from build123d import *

# Parameters (mm, degrees)
SKETCH_1_W          = 40
SKETCH_1_H          = 20
SKETCH_1_R          = 1
EXTRUDE_1_DEPTH     = 40
FILLET_1_R          = 1.5
SKETCH_3_R          = 6.5
EXTRUDE_3_DEPTH     = 1.4
EXTRUDE_START       = 1.4
SKETCH_4_R          = 6.5
EXTRUDE_4_DEPTH     = 1.4
SKETCH_6_R          = 3
EXTRUDE_6_DEPTH     = 4
SKETCH_7_W          = 8
SKETCH_7_H          = 4.7
CUT_EXTRUDE_1_DEPTH = 3
SKETCH_8_W          = 4.7
SKETCH_8_H          = 8
CUT_EXTRUDE_2_DEPTH = 3


with BuildPart() as part:
    # 草图1 → 凸台-拉伸1 (new body)
    with BuildSketch(Plane.XY):
        with Locations((-36.575311459, 110.529011993)):
            Rectangle(SKETCH_1_W, SKETCH_1_H)
        with Locations((-54.575311459, 118.529011993)):
            Circle(SKETCH_1_R, mode=Mode.SUBTRACT)
        with Locations((-54.575311459, 102.529011993)):
            Circle(SKETCH_1_R, mode=Mode.SUBTRACT)
        with Locations((-18.575311459, 102.529011993)):
            Circle(SKETCH_1_R, mode=Mode.SUBTRACT)
        with Locations((-18.575311459, 118.529011993)):
            Circle(SKETCH_1_R, mode=Mode.SUBTRACT)
    extrude(amount=EXTRUDE_1_DEPTH)

    # 圆角1
    fillet_1_edges = [part.edges().sort_by_distance(p)[0] for p in [
        (-16.575311459, 100.529011993, 20),
        (-56.575311459, 100.529011993, 20),
        (-56.575311459, 120.529011993, 20),
        (-16.575311459, 120.529011993, 20),
    ]]
    fillet(fillet_1_edges, radius=FILLET_1_R)

    # 草图3 → 凸台-拉伸3 (add)
    with BuildSketch(Plane.XY.offset(40)):
        with Locations((-46.775311459, 110.529011993)):
            Circle(SKETCH_3_R)
    extrude(amount=EXTRUDE_3_DEPTH)

    # 草图4 → 凸台-拉伸4 (add)
    with BuildSketch(Plane(origin=(0, 0, 0), x_dir=(-1, 0, 0), z_dir=(0, 0, -1)).offset(EXTRUDE_START)):
        with Locations(Location((46.775311459, 110.529011993, 0), (0, 0, 180))):
            Circle(SKETCH_4_R)
    extrude(amount=-EXTRUDE_4_DEPTH)

    # 草图6 → 凸台-拉伸6 (add)
    with BuildSketch(Plane.XY.offset(41.4)):
        with Locations((-46.775311459, 110.529011993)):
            Circle(SKETCH_6_R)
    extrude(amount=EXTRUDE_6_DEPTH)

    # 草图7 → 切除-拉伸1 (cut)
    with BuildSketch(Plane.XZ.offset(-100.529011993)):
        with Locations((-42.575311459, 8.35)):
            Rectangle(SKETCH_7_W, SKETCH_7_H)
    cut_extrude_1 = extrude(amount=-CUT_EXTRUDE_1_DEPTH, mode=Mode.SUBTRACT)

    # 镜向1: 切除-拉伸1 across plane
    add(cut_extrude_1.mirror(Plane(origin=(0, 110.529011993, 0), x_dir=(0, 0, 1), z_dir=(0, -1, 0))), mode=Mode.SUBTRACT)

    # 草图8 → 切除-拉伸2 (cut)
    with BuildSketch(Plane.ZY.offset(56.575311459)):
        with Locations((8.35, 110.529011993)):
            Rectangle(SKETCH_8_W, SKETCH_8_H)
    extrude(amount=-CUT_EXTRUDE_2_DEPTH, mode=Mode.SUBTRACT)


solid = part.part
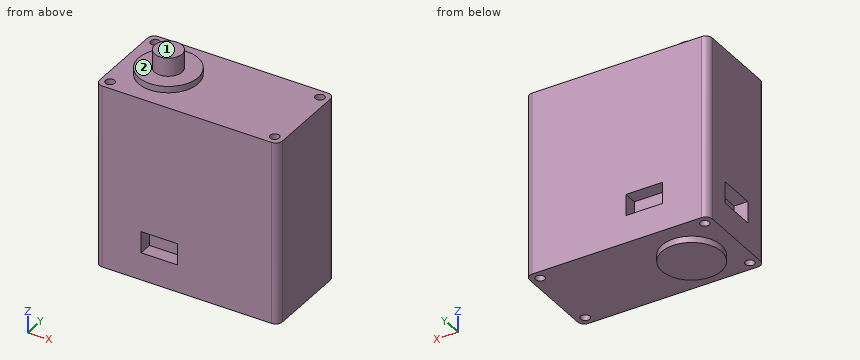
Read the model definition and answer for the solid it produces. Units are mm, in the model's axes. Face numbers are marked on the shaded views. A direction names the side the tool comes from. Give positions to 0.01 mm unless a question says otherwise; leave off trailing zeros. Loops run counter-clockwise (first coordinate to the right, second up) from the corner with the lowest first, then second, coordinate; pieces in that order, holes last. Notation, with made-up numbers: (-5.75, -34.75) -> (11.25, -34.75) arc R20 cw to (11.25, 4.25) -> close; hole circle Ø10 at (84, 61). An arc over 180 degrees is marked (long way). Use a Markdown table: item, result.
Q1. Section D-D, the plane z = 8 is taken. Determine the outline of the cut face in (x, y).
Solved:
| item | result |
|---|---|
| outline | (-56.58, 102.03) arc R1.5 ccw to (-55.08, 100.53) -> (-46.58, 100.53) -> (-46.58, 103.53) -> (-38.58, 103.53) -> (-38.58, 100.53) -> (-18.08, 100.53) arc R1.5 ccw to (-16.58, 102.03) -> (-16.58, 119.03) arc R1.5 ccw to (-18.08, 120.53) -> (-38.58, 120.53) -> (-38.58, 117.53) -> (-46.58, 117.53) -> (-46.58, 120.53) -> (-55.08, 120.53) arc R1.5 ccw to (-56.58, 119.03) -> (-56.58, 114.53) -> (-53.58, 114.53) -> (-53.58, 106.53) -> (-56.58, 106.53) -> close; hole circle Ø2 at (-54.58, 102.53); hole circle Ø2 at (-54.58, 118.53); hole circle Ø2 at (-18.58, 102.53); hole circle Ø2 at (-18.58, 118.53) |
Q2. Section A-A, the plane z = 34 is taken. Determine the outline of the cut face in (x, y), then the cut area to 4 significant figures.
Solved:
| item | result |
|---|---|
| outline | (-56.58, 102.03) arc R1.5 ccw to (-55.08, 100.53) -> (-18.08, 100.53) arc R1.5 ccw to (-16.58, 102.03) -> (-16.58, 119.03) arc R1.5 ccw to (-18.08, 120.53) -> (-55.08, 120.53) arc R1.5 ccw to (-56.58, 119.03) -> close; hole circle Ø2 at (-54.58, 102.53); hole circle Ø2 at (-54.58, 118.53); hole circle Ø2 at (-18.58, 102.53); hole circle Ø2 at (-18.58, 118.53) |
| area | 785.5 mm^2 |
Q3. Section B-B, the plane x = -48 is taken. Determine the outline of the cut face in (y, z), then the cut area to 3 significant figures.
Solved:
| item | result |
|---|---|
| outline | (100.53, 0) -> (104.15, 0) -> (104.15, -1.4) -> (116.91, -1.4) -> (116.91, 0) -> (120.53, 0) -> (120.53, 40) -> (116.91, 40) -> (116.91, 41.4) -> (113.27, 41.4) -> (113.27, 45.4) -> (107.79, 45.4) -> (107.79, 41.4) -> (104.15, 41.4) -> (104.15, 40) -> (100.53, 40) -> close |
| area | 858 mm^2 |
Q4. Each of these flat-tipped pins is pushed along its axis until it touches: pin 1 (3.5 mm diameter, centred on x = -55.5, y = 109.5, fed in from +Z); pin 2 (3.5 mm diameter, centred on x = -41, y = 119, fed in from -Z); pin 3 (4 mm diameter, centred on x = -44.5, z = 8.5, fed in from -Y); pin 4 (10.5 mm diameter, centred on x = -45, y = 113.5, fed in from +Z). Where does it stop, or does it pass through?
Solved:
| item | result |
|---|---|
| pin 1 | stops at z = 40 |
| pin 2 | stops at z = 0 |
| pin 3 | stops at y = 103.53 |
| pin 4 | stops at z = 45.4 |
Q5. Find the intervals of material crossed by line 1 along X through (y, z) = (118.5, 7); line 2 along Y through (x, z) = (-54, 7.5); line 3 along Z through (x, y) = (-23.5, 109.25), in increasing order.
Solved:
| item | result |
|---|---|
| line 1 | x = -56.58 to -55.57, -53.58 to -46.58, -38.58 to -19.57, -17.58 to -16.58 |
| line 2 | y = 100.53 to 101.71, 103.35 to 106.53, 114.53 to 117.71, 119.35 to 120.53 |
| line 3 | z = 0 to 40 |
Q6. A tool of negligible diameter and unlimited length cuts with its end or side. For the marked faces 1 and 2, from which of +Z, -Z, +X, -X, +Y, -Y can it reach the whole face along a straight path? Write none if from no direction.
Solved:
| item | result |
|---|---|
| face 1 | +Z, +X, -X, +Y, -Y |
| face 2 | +Z |
Q7. Section C-C, the plane y = 112.5 is taken. Determine the outline of the cut face in (x, z), then the cut area to 3 significant figures.
Solved:
| item | result |
|---|---|
| outline | (-56.58, 0) -> (-52.97, 0) -> (-52.97, -1.4) -> (-40.58, -1.4) -> (-40.58, 0) -> (-16.58, 0) -> (-16.58, 40) -> (-40.58, 40) -> (-40.58, 41.4) -> (-44.51, 41.4) -> (-44.51, 45.4) -> (-49.04, 45.4) -> (-49.04, 41.4) -> (-52.97, 41.4) -> (-52.97, 40) -> (-56.58, 40) -> (-56.58, 10.7) -> (-53.58, 10.7) -> (-53.58, 6) -> (-56.58, 6) -> close |
| area | 1,640 mm^2 |
